Geometry: final body of the model. Coordinates: model frame, mm. Face numbers are marked on the shaded views. Give positions to 0.01 mm unless a question says otherwise; leave off trailing zeros. Loops run counter-clockwise (first coordinate to the right, second up) from the corner with the lowest first, then second, coordinate; pieces in that order, holes last. Notation, with made-up numbers: (27.25, 73) -> (80.25, 73) arc R14 cw to (80.25, 87) -> close; hole circle Ø8 at (47.5, 75.5). An arc over 180 degrees is marked (long way). One line per question, with ' | ' between items. Start each with the question number.
Item 1: Pin query (flat end, axial travel): P1, Ø1.5, axis at x = -14, z = 5, coming from the -Y side; P2, Ø2, axis at y = 5, z = 1, coming from the +X side; P3, Ø12, axis at x = -7.5, y = -13.5, coming from the -Z side; P4, Ø10, axis at x = -3.5, y = 7, coming from the +Z side. Return the tip coordinate at first contact, or that it passes through.
Item 2: Section A-A on y = 0. Return loops of the section in (x, z).
Item 3: Material intervals for line 1 along Y through (x, z) = (0, 2.95); line 2 along X through (y, z) = (-0.5, 0.8); line 3 along X through (y, z) = (-11.5, 4.7), sorted ascending. Write a range as [from, to].
Item 4: Section B-B on x = 0. Return loops of the section in (y, z).
Item 5: Mould query, pull axis Y, two halves, no side actions, for the marked faces 1, 2 and 3. Classes: released by +Y, released by -Y, zero draft, split by the parting line, or undercut.
Item 6: Section C-C on z = 4.25. Return loops of the section in (x, y).
Autodesk Inventor part; units mm, degrees
ref_plane "YZ Plane" through (0, 0, 0) normal (1, 0, 0) x (0, 1, 0)
ref_plane "XZ Plane" through (0, 0, 0) normal (0, 1, 0) x (-1, 0, 0)
ref_plane "XY Plane" through (0, 0, 0) normal (0, 0, 1) x (1, 0, 0)
sketch "Sketch1" plane through (0, 0, 0) normal (0, 0, 1) x (1, 0, 0)
  circle A0 centre (0, 0) radius 16
  circle A1 centre (0, 0) radius 20
  dimension "d0" = 32
  dimension "d1" = 40
extrude "Extrusion1" add sketch "Sketch1" along normal blind 6
sketch "Sketch2" plane through (0, 0, 6) normal (0, 0, 1) x (1, 0, 0)
  line L0 (-4.3061, 18.5) -> (4.6939, 18.5) construction
  line L1 (-4.5, 20) -> (4.5, 20) construction
  circle A0 centre (0, 0) radius 20 construction
  circle A1 centre (0, 0) radius 20
  arc A2 (4.8649, 19.3993) -> (-4.8649, 19.3993) centre (0, 0) ccw
  arc A3 (4.5, 17.9444) -> (-4.5, 17.9444) centre (0, 0) ccw
  line L2 (4.5, 17.9444) -> (4.8649, 19.3993)
  line L3 (-4.5, 17.9444) -> (-4.8649, 19.3993)
  line L4 (-4.8649, 19.3993) -> (0, 0) construction
  line L5 (4.8649, 19.3993) -> (0, 0) construction
  circle A4 centre (0, 0) radius 16 construction
  line L6 (-16, 0) -> (16, 0) construction
  arc A5 (-4.8649, -19.3993) -> (4.8649, -19.3993) centre (0, 0) ccw
  arc A6 (-4.5, -17.9444) -> (4.5, -17.9444) centre (0, 0) ccw
  line L7 (4.5, -17.9444) -> (4.8649, -19.3993)
  line L8 (-4.5, -17.9444) -> (-4.8649, -19.3993)
  point P0 (0, 20)
  point P1 (0, -20)
  dimension "d4" = 9
  dimension "d5" = 1.5
extrude "Extrusion2" cut sketch "Sketch2" against normal through all contours L2 A3 L3 A1 | A1 L8 A6 L7
equation "\"d1\" = BattECOD"
equation "\"d5\" = GripLength"
properties part number "Battery Tube Collar"
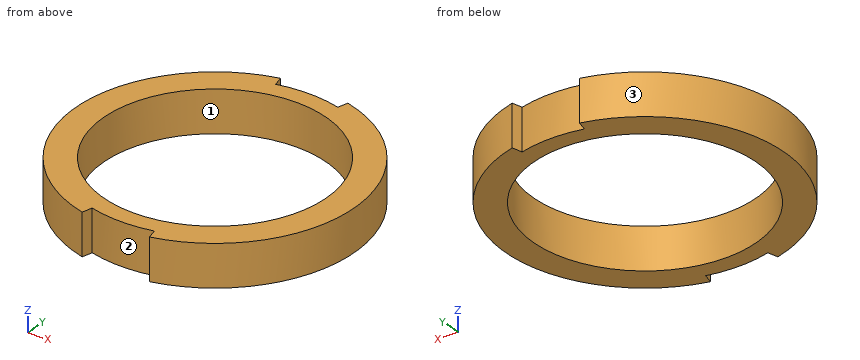
Result sheet:
1) P1: stops at y = -14.98 | P2: stops at x = 19.6 | P3: stops at z = 0 | P4: passes through
2) outline: (-20, 0) -> (-16, 0) -> (-16, 6) -> (-20, 6) -> close; (16, 0) -> (20, 0) -> (20, 6) -> (16, 6) -> close
3) line 1: y = [-18.5, -16], [16, 18.5] | line 2: x = [-19.99, -15.99], [15.99, 19.99] | line 3: x = [-16.36, -11.12], [11.12, 16.36]
4) outline: (-18.5, 0) -> (-16, 0) -> (-16, 6) -> (-18.5, 6) -> close; (16, 0) -> (18.5, 0) -> (18.5, 6) -> (16, 6) -> close
5) face 1: undercut | face 2: released by -Y | face 3: split by the parting line
6) outline: (-4.86, -19.4) -> (-4.5, -17.94) arc R18.5 ccw to (4.5, -17.94) -> (4.86, -19.4) arc R20 ccw to (4.86, 19.4) -> (4.5, 17.94) arc R18.5 ccw to (-4.5, 17.94) -> (-4.86, 19.4) arc R20 ccw to start; hole circle Ø32 at (0, 0)
